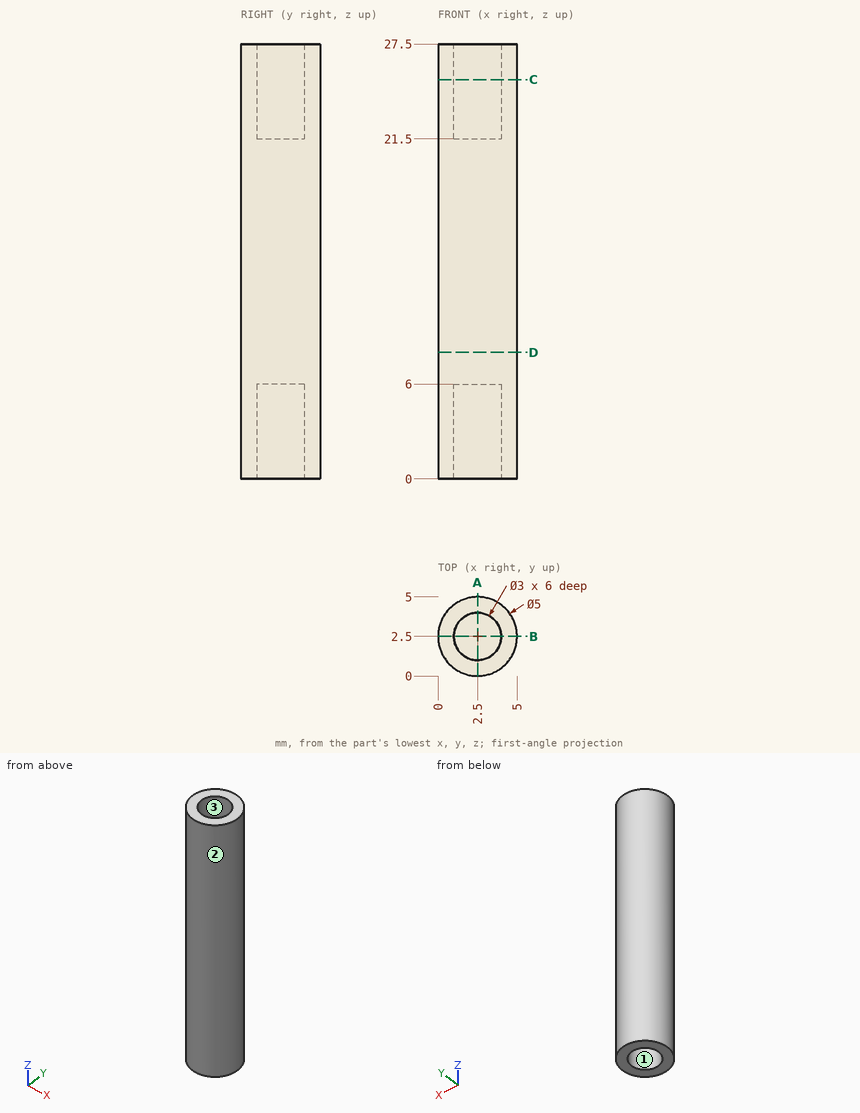
Study the drawing (mm; zero at the part's minimum x, y, z) and answer. Give positions to 0.01 mm unless a question says otherwise; leave off trailing zeros. Loops run counter-clockwise (first coordinate to the right, second up) from the corner with the lowest first, then second, coordinate; pieces in that order, holes last. Notation, with made-up numbers: M 56.5,-30 L 86.5,-30 A27 ccw 86.5,-2 Z; hole C 50.5,-5 d1. An arc over 180 degrees is marked long. Answer as CSV lines item,"result".
Item 1: Straight lines are drawn through the part: line 1 along Y through (x, z) = (2.5, 2.3); line 2 along Y through (x, z) = (0.5, 10.5); line 3 along Z through (x, y) = (1.1, 2.65). For each, find the intervals that lie inside material, in ascending order. Write a range as [from, to].
Values follow:
line 1,"y = [0, 1], [4, 5]"
line 2,"y = [1, 4]"
line 3,"z = [6, 21.5]"
Item 2: Given pin 1 Ø2.5 at (x, y) = (2.5, 2.5) entering from +Z; pin 2 Ø2 at (x, z) = (0.5, 23.5) entering from +Y; pin 3 Ø2.5 at (x, y) = (2.5, 2.5) entering from -Z, each flat-ended and moving along its own axis, determine where each tip first touches the part or whether it passes through.
Values follow:
pin 1,"stops at z = 21.5"
pin 2,"stops at y = 4.79"
pin 3,"stops at z = 6"
Item 3: The part is cut by section A-A (x = 2.5). Give the vertices of the cut face in (y, z), and give its area (4 significant figures).
Values follow:
outline,"M 0,0 L 1,0 L 1,6 L 4,6 L 4,0 L 5,0 L 5,27.5 L 4,27.5 L 4,21.5 L 1,21.5 L 1,27.5 L 0,27.5 Z"
area,"101.5 mm^2"
Item 4: The part is cut by section C-C (z = 25.25). Give the vertices of the cut face in (x, y), and give its area (3 significant figures).
Values follow:
outline,"C 2.5,2.5 d5; hole C 2.5,2.5 d3"
area,"12.6 mm^2"
Item 5: The part is cut by section D-D (z = 8). Give the vertices of the cut face in (x, y).
Values follow:
outline,"C 2.5,2.5 d5"
Item 6: The mould has two halves that part along Y. Classify the marked faces 1, 2 and 3: released by +Y, released by -Y, zero draft, split by the parting line, or undercut.
Values follow:
face 1,"undercut"
face 2,"split by the parting line"
face 3,"undercut"
